Part model, mm, in its own coordinate system. Face numbers are marked on the shaded views. A direction names the side the tool comes from. Give positions to 0.01 mm unless a question says otherwise; leave off trailing zeros. Order: outer loops, then holes, each group sorted by start corner. A loop starts at its lowest first (then second) coordinate and runs counter-clockwise, first axis right, second up. Notation, with made-up numbers: (45.5, -15) -> (90.5, -15) arc R14 ccw to (90.5, -7) -> close; hole circle Ø1 at (71, 55). An arc over 180 degrees is marked (long way). Write item = value, one per line. Start each with the question number.
Item 1: Band-saw the part on B-B on z = 28. Write the cut outline in (x, y).
Item 2: Tool access for the marked faces 1 and 2: list every direction of +Z, -Z, +X, -X, +Y, -Y with a clear straight run to the whole face (end or side of a thin tool).
Item 3: Band-saw the part on C-C on x = -15. Write the cut outline in (y, z).
Item 4: Band-saw the part on A-A on y = -3. Write the cut outline in (x, z), plus the area to 3 significant figures.
Item 5: Band-saw the part on D-D on y = -28. Write the cut outline in (x, z).
Item 6: Drill centre lines: line 1 along X through (y, z) = (-24.5, 14); line 2 along Y through (x, z) = (38, -31.5); line 3 along X through (y, z) = (-18, -4.5). Where is each one in solid material? Low to high.
Item 7: Flat gauge pin, fed straight in: P1, Ø8, axis at x = -24, z = 6, coming from the +Y side. Where does the tip first touch, or does it go through?
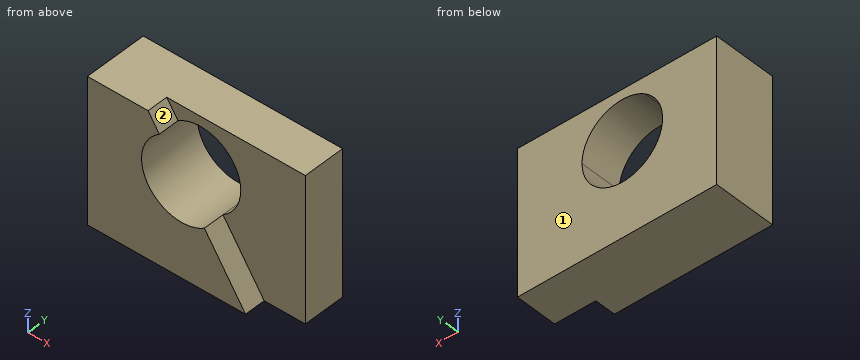
```python
from build123d import *

# Parameters (mm, degrees)
F1_DEPTH = 38.1
F2_DEPTH = 25.4


with BuildPart() as f1:
    # F0 (on Front) → F1 (new body)
    with BuildSketch(Plane.XZ):
        with BuildLine():
            Line((-16.724718, 33.538792), (-23.510048, 43.607347))
            Line((-23.510048, 43.607347), (-60.102299, 43.607347))
            Line((-60.102299, 43.607347), (-60.102299, -43.607347))
            Line((-60.102299, -43.607347), (35.265073, -43.607347))
            Line((35.265073, -43.607347), (10.436524, -6.764985))
            ThreePointArc((10.436524, -6.764985), (-23.295985, -0.193718), (-16.724718, 33.538792))
        make_face()
    extrude(amount=F1_DEPTH)

    # F0 (on Front) → F2 (join)
    with BuildSketch(Plane.XZ):
        with BuildLine():
            Line((60.102299, -43.607347), (60.102299, 43.607347))
            Line((60.102299, 43.607347), (-23.510048, 43.607347))
            Line((-23.510048, 43.607347), (-16.724718, 33.538792))
            ThreePointArc((-16.724718, 33.538792), (8.268859, 34.840955), (21.156765, 13.386903))
            ThreePointArc((21.156765, 13.386903), (18.309955, 1.973948), (10.436524, -6.764985))
            Line((10.436524, -6.764985), (35.265073, -43.607347))
            Line((35.265073, -43.607347), (60.102299, -43.607347))
        make_face()
    extrude(amount=F2_DEPTH)


solid = f1.part
```
Values found:
q1.outline = (-60.1, -38.1) -> (-22.56, -38.1) -> (-22.56, 0) -> (-60.1, 0) -> close; (16.27, -25.4) -> (60.1, -25.4) -> (60.1, 0) -> (16.27, 0) -> close
q2.face_1 = +Z, -Z, +X, -X, +Y
q2.face_2 = +Z, +X, -Y
q3.outline = (-38.1, -43.61) -> (0, -43.61) -> (0, -7.83) -> (-38.1, -7.83) -> close; (-25.4, 34.6) -> (0, 34.6) -> (0, 43.61) -> (-25.4, 43.61) -> close
q4.outline = (-60.1, -43.61) -> (60.1, -43.61) -> (60.1, 43.61) -> (-60.1, 43.61) -> close; hole (10.44, -6.76) arc R24.3 ccw to (21.16, 13.39) arc R24.3 ccw (long way) to start
q4.area = 8,630 mm^2
q5.outline = (-60.1, -43.61) -> (35.27, -43.61) -> (10.44, -6.76) arc R24.3 cw to (-16.72, 33.54) -> (-23.51, 43.61) -> (-60.1, 43.61) -> close
q6.line_1 = -60.1 to -27.44, 21.15 to 60.1
q6.line_2 = -25.4 to 0
q6.line_3 = -60.1 to -19.59, 13.31 to 60.1
q7.P1 = 0
